```python
from build123d import *

# Parameters (mm, degrees)
F0_W     = 12
F0_H     = 30
F1_DEPTH = 6
F2_DEPTH = 6


with BuildPart() as f1:
    # F0 (on Right) → F1 (new body, symmetric)
    with BuildSketch(Plane.YZ):
        Polygon((0, 30), (0, 0), (90, 0), (180, 0), (180, 30), (180, 60), (180, 90), (90, 90), (0, 90), (0, 60), align=None)
        with Locations((-6, 45)):
            Rectangle(F0_W, F0_H)
        with Locations((186, 45)):
            Rectangle(F0_W, F0_H)
    extrude(amount=F1_DEPTH, both=True)

    # F0 (on Right) → F2 (join, symmetric)
    with BuildSketch(Plane.YZ):
        Polygon((0, 30), (0, 0), (90, 0), (180, 0), (180, 30), (180, 60), (180, 90), (90, 90), (0, 90), (0, 60), align=None)
        with Locations((-6, 45)):
            Rectangle(F0_W, F0_H)
        with Locations((186, 45)):
            Rectangle(F0_W, F0_H)
    extrude(amount=F2_DEPTH, both=True)


solid = f1.part
```
Source: CAD feature listing. Evaluate the final solid. Frame: model axes, mm. A direction names the side the tool comes from. Coordinates: 2 decimals unless noted, no trailing zeros. Loops run counter-clockwise (first coordinate to the right, second up) from the corner with the lowest first, then second, coordinate; pieces in that order, holes last. Notation, with made-up numbers: M 37,-31.75 L 72,-31.75 A29 cw 72,1.25 Z; hole C 44,38.5 d10. An arc over 180 degrees is marked long. Use CSV: the item, a comma, the result in double quotes.
(1) Line query: line 1 (Y direction, x = -0.25, z = 69). Output: solid intervals per line, ascending. Write a range as [from, to].
Answers follow:
line 1,"[0, 180]"
(2) Contact query for flat-ended pins moving along their axis: pin 1 (3.5 mm diameter, centred on x = -1, z = 69, fed in from +Y); pin 2 (3.5 mm diameter, centred on x = 2, y = 188, fed in from -Z); pin 3 (6 mm diameter, centred on x = -0.5, z = 82.5, fed in from -Y). Output: stop coordinate, or through.
Answers follow:
pin 1,"y = 180"
pin 2,"z = 30"
pin 3,"y = 0"
(3) Cut plane B-B on z = 82. Return loops of the section in (x, y), and give its area (3 significant figures).
Answers follow:
outline,"M -6,0 L 6,0 L 6,180 L -6,180 Z"
area,"2,160 mm²"
(4) Cut plane A-A on x = 4. Return loops of the section in (y, z), and give its area (3 significant figures).
Answers follow:
outline,"M -12,30 L 0,30 L 0,0 L 180,0 L 180,30 L 192,30 L 192,60 L 180,60 L 180,90 L 0,90 L 0,60 L -12,60 Z"
area,"16,900 mm²"
(5) Reachability of faces 1 (the face through (0, 180, 15)), 2 (the face through (0, -6, 30)), 3 (the face through (0, 180, 75)) from +Z, -Z, +X, -X, +Y, -Y: full face, straight path, thin tool, end or side. Return the list, or none.
Answers follow:
face 1,"-Z, +X, -X, +Y"
face 2,"-Z, +X, -X, -Y"
face 3,"+Z, +X, -X, +Y"
